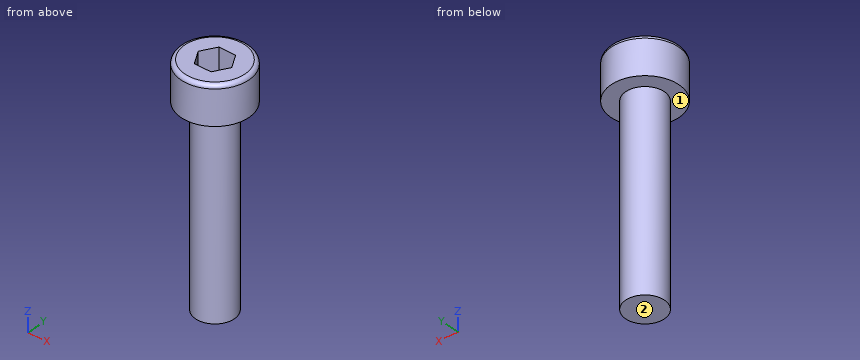
Solid Edge part; units mm, degrees
sketch "Sketch1" plane through (0, 0, 0) normal (0, 0, 1) x (1, 0, 0)
  circle A0 centre (0, 0) radius 1
extrude "Protrusion1" add sketch "Sketch1" along normal blind 10
sketch "Sketch2" plane through (0, 0, 10) normal (0, 0, 1) x (1, 0, 0)
  circle A0 centre (0, 0) radius 1.75
extrude "ExtrudedProtrusion_2" add sketch "Sketch2" along normal blind 2
sketch "Sketch3" plane through (0, 0, 12) normal (0, 0, 1) x (1, 0, 0)
  line L0 (0.433, 0.75) -> (0.866, 0)
  line L1 (0.866, 0) -> (0.433, -0.75)
  line L2 (0.433, -0.75) -> (-0.433, -0.75)
  line L3 (-0.433, -0.75) -> (-0.866, 0)
  line L4 (-0.866, 0) -> (-0.433, 0.75)
  line L5 (-0.433, 0.75) -> (0.433, 0.75)
extrude "ExtrudedCutout_1" cut sketch "Sketch3" against normal blind 1.5
fillet "Round_1" radius 0.2 1 edges at (-1.75, 0, 12)
cosmetic_thread "Thread1"
Could you check a few things on this model? Use its own coordinates, in mm. Face numbers are marked on the shaded views. A direction names the side the tool comes from. Give positions to 0.01 mm unless a question says otherwise; leave off trailing zeros. Loops run counter-clockwise (first coordinate to the right, second up) from the corner with the lowest first, then second, coordinate; pieces in that order, holes last. Notation, with made-up numbers: (78, 37.5) -> (130, 37.5) arc R19 ccw to (130, 42.5) -> close; hole circle Ø10 at (75, 82). An arc over 180 degrees is marked (long way). Return JSON: item names as keys, results as strings.
Item 1: I'm going to push flat-ended pins straight in: pin 1 (2 mm diameter, centred on x = 1, z = 6.5, fed in from +Y); pin 2 (2 mm diameter, centred on y = -1, z = 4, fed in from +X). Where does each tip first touch, or does it pass through?
Geometry results:
{"pin 1": "stops at y = 1", "pin 2": "stops at x = 1"}
Item 2: Which directions (+Z, -Z, +X, -X, +Y, -Y) give clear straight access to the entire face, cutting with the end or side of a thin tool? Please do the marked faces 1 and 2.
Geometry results:
{"face 1": "-Z", "face 2": "-Z, +X, -X, +Y, -Y"}
Item 3: I need wall thicknesses on L1, parallel to Y at x = 0, z = 10.75; L2, parallel to Z at x = 1.25, y = 0.65; L3, parallel to Z at x = 0.2, y = 0.65. Which ranges of each line are inside material? Lowest first, please. Write a range as from..to.
Geometry results:
{"L1": "y = -1.75..-0.75, 0.75..1.75", "L2": "z = 10..12", "L3": "z = 0..10.5"}
Item 4: If we section it at A-A on x = 0: List the corners of the cut face in (y, z) for me.
Geometry results:
{"outline": "(-1.75, 10) -> (-1, 10) -> (-1, 0) -> (1, 0) -> (1, 10) -> (1.75, 10) -> (1.75, 11.8) arc R0.2 ccw to (1.55, 12) -> (0.75, 12) -> (0.75, 10.5) -> (-0.75, 10.5) -> (-0.75, 12) -> (-1.55, 12) arc R0.2 ccw to (-1.75, 11.8) -> close"}
Item 5: If we section it at B-B on z = 8.5: List the corners of the cut face in (x, y) for me.
Geometry results:
{"outline": "circle Ø2 at (0, 0)"}
